Drawing for the job (mm, zero at the part's lowest x, y, z). Round coordinates to 2 decimals unless told otherwise and drop trailing zeros. Loops run counter-clockwise (first coordinate to the right, second up) from the corner with the lowest first, then second, coordinate; pieces in that order, holes last. Notation, with made-up numbers: (-28.75, -2.75) - (10.25, -2.75) arc R10 ccw to (10.25, 15.25) - close; hole circle Ø11 at (-10.75, 4.5). An arc over 180 degrees is marked (long way). Put each result on its own line as item: value.
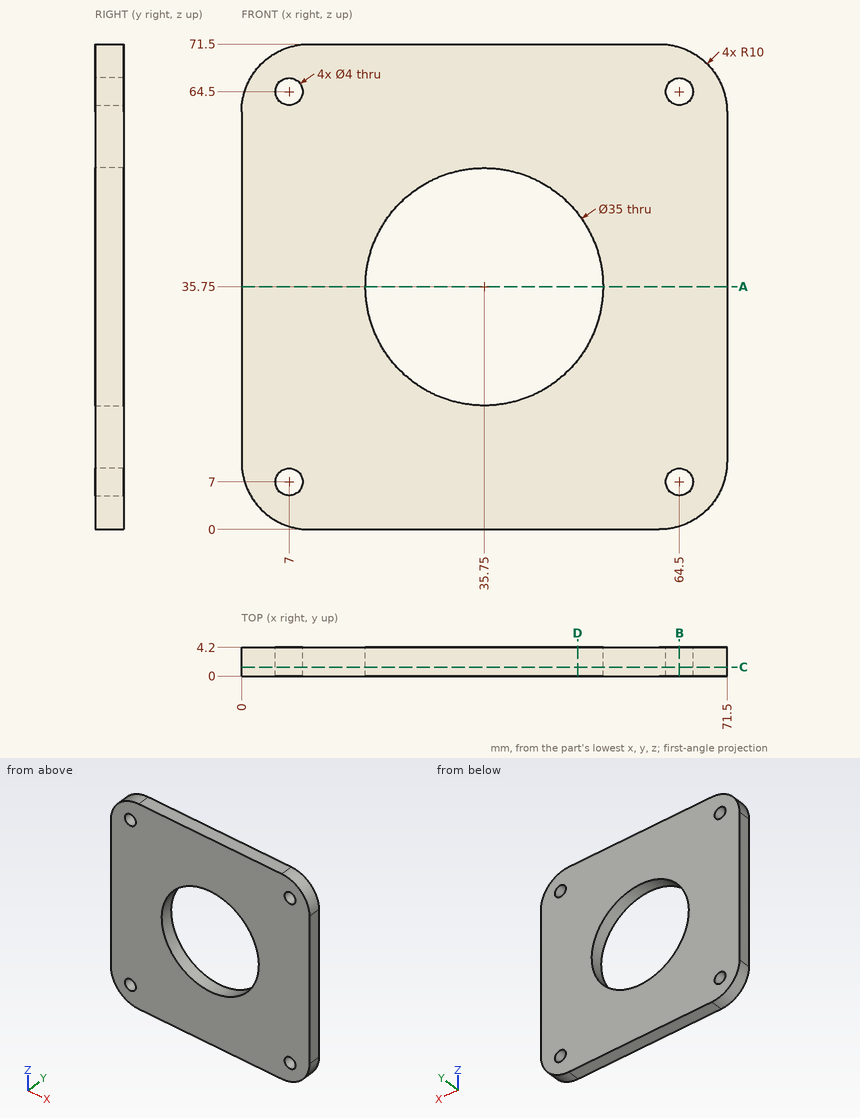
1. Band-saw the part on A-A (z = 35.75). List the corners of the cut face in (x, y).
A:
outline: (0, 0) - (18.25, 0) - (18.25, 4.2) - (0, 4.2) - close; (53.25, 0) - (71.5, 0) - (71.5, 4.2) - (53.25, 4.2) - close
2. Band-saw the part on D-D (x = 49.5). List the corners of the cut face in (y, z), plus the area to 3 significant figures.
A:
outline: (0, 0) - (4.2, 0) - (4.2, 24.92) - (0, 24.92) - close; (0, 46.58) - (4.2, 46.58) - (4.2, 71.5) - (0, 71.5) - close
area: 209 mm²
3. Band-saw the part on B-B (x = 64.5). List the corners of the cut face in (y, z).
A:
outline: (0, 0.46) - (4.2, 0.46) - (4.2, 5) - (0, 5) - close; (0, 9) - (4.2, 9) - (4.2, 62.5) - (0, 62.5) - close; (0, 66.5) - (4.2, 66.5) - (4.2, 71.04) - (0, 71.04) - close
4. Band-saw the part on C-C (y = 1.3). List the corners of the cut face in (x, z).
A:
outline: (0, 10) arc R10 ccw to (10, 0) - (61.5, 0) arc R10 ccw to (71.5, 10) - (71.5, 61.5) arc R10 ccw to (61.5, 71.5) - (10, 71.5) arc R10 ccw to (0, 61.5) - close; hole circle Ø4 at (7, 7); hole circle Ø4 at (7, 64.5); hole circle Ø35 at (35.75, 35.75); hole circle Ø4 at (64.5, 7); hole circle Ø4 at (64.5, 64.5)
5. Probe line 1 along Z through (x, y) = (64.5, 2.45); line 2 along X through (y, z) = (2.4, 35.75). List the from-to ranges inside material, lowest first. Write a range as [from, to].
A:
line 1: z = [0.46, 5], [9, 62.5], [66.5, 71.04]
line 2: x = [0, 18.25], [53.25, 71.5]
